Geometry: final body of the model. Coordinates: model frame, mm. Face numbers are marked on the shaded views. A direction names the side the tool comes from. Round coordinates to 2 decimals unless told otherwise and drop trailing zeros. Loops run counter-clockwise (first coordinate to the right, second up) from the corner with the lowest first, then second, coordinate; pieces in that order, holes last. Notation, with made-up numbers: (7, 21) -> (46, 21) arc R9 cw to (46, 27) -> close; hole circle Ø1 at (18.25, 61.25). An arc over 180 degrees is marked (long way). Answer in a Markdown table with one row per item.
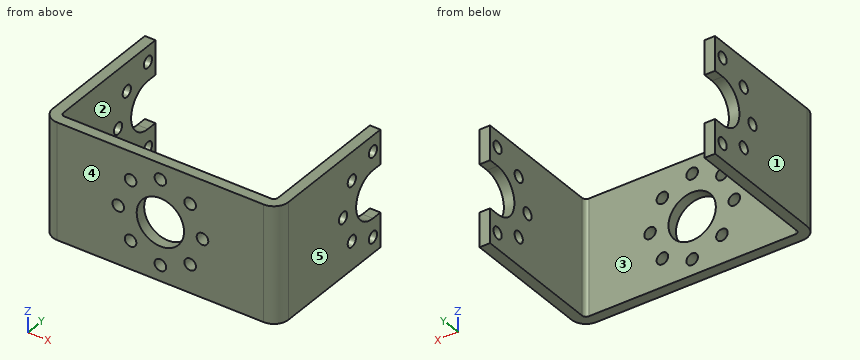
```python
from build123d import *

# Parameters (mm, degrees)
SKETCH_1_R             = 4.5
SKETCH_1_R_2           = 1.1
SM_BASE_FLANGE_1_DEPTH = 2
OTHER_START            = -47
OTHER_1_OUTLINE_W      = 2
OTHER_1_OUTLINE_H      = 22
OTHER_1_DEPTH          = 24.627322451
OTHER_START_2          = 22.372677549
OTHER_1_2_OUTLINE_W    = 2
OTHER_1_2_OUTLINE_H    = 22
OTHER_1_2_DEPTH        = 24.627322451
OTHER_START_3          = -22.106515833
OTHER_1_3_OUTLINE_R    = 1.1
OTHER_1_3_DEPTH        = 1.733838284
OTHER_START_4          = 20.372677549
OTHER_1_4_OUTLINE_R    = 1.1
OTHER_1_4_DEPTH        = 1.733838284
OTHER_START_5          = -22.372677549
OTHER_1_5_OUTLINE_R    = 1.1
OTHER_1_5_DEPTH        = 2.7366
OTHER_START_6          = 19.636077549
OTHER_1_6_OUTLINE_R    = 1.1
OTHER_1_6_DEPTH        = 2.7366
OTHER_START_7          = -12
OTHER_1_7_DEPTH        = 24


with BuildPart() as part:
    # 基体-法兰1: sheet metal written as solids
    # Sketch 1 → 基体-法兰1 (new body)
    with BuildSketch(Plane(origin=(0, 0, 0), x_dir=(1, 0, 0), z_dir=(0, 1, 0))):
        with BuildLine():
            Line((-45, -11), (-47, -11))
            Line((-47, -11), (-47, -4.5))
            Line((-47, -4.5), (-45, -4.5))
            ThreePointArc((-45, -4.5), (-40.5, 0), (-45, 4.5))
            Line((-45, 4.5), (-47, 4.5))
            Line((-47, 4.5), (-47, 11))
            Line((-47, 11), (-45, 11))
            Line((-45, 11), (45, 11))
            Line((45, 11), (47, 11))
            Line((47, 11), (47, 4.5))
            Line((47, 4.5), (45, 4.5))
            ThreePointArc((45, 4.5), (40.5, 0), (45, -4.5))
            Line((45, -4.5), (47, -4.5))
            Line((47, -4.5), (47, -11))
            Line((47, -11), (45, -11))
            Line((45, -11), (-45, -11))
        make_face()
        with Locations(Location((0, 0, 0), (0, 0, 270))):
            Circle(SKETCH_1_R, mode=Mode.SUBTRACT)
        with Locations(Location((0, 8, 0), (0, 0, 270))):
            Circle(SKETCH_1_R_2, mode=Mode.SUBTRACT)
        with Locations(Location((5.656854249, 5.656854249, 0), (0, 0, 270))):
            Circle(SKETCH_1_R_2, mode=Mode.SUBTRACT)
        with Locations(Location((8, 0, 0), (0, 0, 270))):
            Circle(SKETCH_1_R_2, mode=Mode.SUBTRACT)
        with Locations(Location((5.656854249, -5.656854249, 0), (0, 0, 270))):
            Circle(SKETCH_1_R_2, mode=Mode.SUBTRACT)
        with Locations(Location((0, -8, 0), (0, 0, 270))):
            Circle(SKETCH_1_R_2, mode=Mode.SUBTRACT)
        with Locations(Location((-5.656854249, -5.656854249, 0), (0, 0, 270))):
            Circle(SKETCH_1_R_2, mode=Mode.SUBTRACT)
        with Locations(Location((-8, 0, 0), (0, 0, 270))):
            Circle(SKETCH_1_R_2, mode=Mode.SUBTRACT)
        with Locations(Location((-5.656854249, 5.656854249, 0), (0, 0, 270))):
            Circle(SKETCH_1_R_2, mode=Mode.SUBTRACT)
        with Locations(Location((-45, 8, 0), (0, 0, 270))):
            Circle(SKETCH_1_R_2, mode=Mode.SUBTRACT)
        with Locations(Location((-39.343145751, 5.656854249, 0), (0, 0, 270))):
            Circle(SKETCH_1_R_2, mode=Mode.SUBTRACT)
        with Locations(Location((-37, 0, 0), (0, 0, 270))):
            Circle(SKETCH_1_R_2, mode=Mode.SUBTRACT)
        with Locations(Location((-39.343145751, -5.656854249, 0), (0, 0, 270))):
            Circle(SKETCH_1_R_2, mode=Mode.SUBTRACT)
        with Locations(Location((-45, -8, 0), (0, 0, 270))):
            Circle(SKETCH_1_R_2, mode=Mode.SUBTRACT)
        with Locations(Location((45, 8, 0), (0, 0, 270))):
            Circle(SKETCH_1_R_2, mode=Mode.SUBTRACT)
        with Locations(Location((45, -8, 0), (0, 0, 270))):
            Circle(SKETCH_1_R_2, mode=Mode.SUBTRACT)
        with Locations(Location((39.343145751, -5.656854249, 0), (0, 0, 270))):
            Circle(SKETCH_1_R_2, mode=Mode.SUBTRACT)
        with Locations(Location((37, 0, 0), (0, 0, 270))):
            Circle(SKETCH_1_R_2, mode=Mode.SUBTRACT)
        with Locations(Location((39.343145751, 5.656854249, 0), (0, 0, 270))):
            Circle(SKETCH_1_R_2, mode=Mode.SUBTRACT)
    extrude(amount=-SM_BASE_FLANGE_1_DEPTH)

    # Other 1: read off the stored shape, not the designer's step
    # Other 1 outline → Other 1 (cut)
    with BuildSketch(Plane.YZ.offset(OTHER_START)):
        with Locations((-1, 0)):
            Rectangle(OTHER_1_OUTLINE_W, OTHER_1_OUTLINE_H)
    extrude(amount=OTHER_1_DEPTH, mode=Mode.SUBTRACT)

    # Other 1 2 outline → Other 1 2 (cut)
    with BuildSketch(Plane.YZ.offset(OTHER_START_2)):
        with Locations((-1, 0)):
            Rectangle(OTHER_1_2_OUTLINE_W, OTHER_1_2_OUTLINE_H)
    extrude(amount=OTHER_1_2_DEPTH, mode=Mode.SUBTRACT)

    # Other 1 3 outline → Other 1 3 (add)
    with BuildSketch(Plane.YZ.offset(OTHER_START_3)):
        with BuildLine():
            Line((0, 11), (0, -11))
            Line((0, -11), (25.372677549, -11))
            Line((25.372677549, -11), (25.372677549, -4.5))
            Line((25.372677549, -4.5), (23.372677549, -4.5))
            ThreePointArc((23.372677549, -4.5), (18.872677549, 0), (23.372677549, 4.5))
            Line((23.372677549, 4.5), (25.372677549, 4.5))
            Line((25.372677549, 4.5), (25.372677549, 11))
            Line((25.372677549, 11), (0, 11))
        make_face()
        with Locations((17.7158233, -5.656854249)):
            Circle(OTHER_1_3_OUTLINE_R, mode=Mode.SUBTRACT)
        with Locations((23.372677549, -8)):
            Circle(OTHER_1_3_OUTLINE_R, mode=Mode.SUBTRACT)
        with Locations((15.372677549, 0)):
            Circle(OTHER_1_3_OUTLINE_R, mode=Mode.SUBTRACT)
        with Locations((17.7158233, 5.656854249)):
            Circle(OTHER_1_3_OUTLINE_R, mode=Mode.SUBTRACT)
        with Locations((23.372677549, 8)):
            Circle(OTHER_1_3_OUTLINE_R, mode=Mode.SUBTRACT)
    extrude(amount=OTHER_1_3_DEPTH)

    # Other 1 4 outline → Other 1 4 (add)
    with BuildSketch(Plane.YZ.offset(OTHER_START_4)):
        with BuildLine():
            Line((0, 11), (0, -11))
            Line((0, -11), (25.372677549, -11))
            Line((25.372677549, -11), (25.372677549, -4.5))
            Line((25.372677549, -4.5), (23.372677549, -4.5))
            ThreePointArc((23.372677549, -4.5), (18.872677549, 0), (23.372677549, 4.5))
            Line((23.372677549, 4.5), (25.372677549, 4.5))
            Line((25.372677549, 4.5), (25.372677549, 11))
            Line((25.372677549, 11), (0, 11))
        make_face()
        with Locations((17.7158233, -5.656854249)):
            Circle(OTHER_1_4_OUTLINE_R, mode=Mode.SUBTRACT)
        with Locations((23.372677549, -8)):
            Circle(OTHER_1_4_OUTLINE_R, mode=Mode.SUBTRACT)
        with Locations((15.372677549, 0)):
            Circle(OTHER_1_4_OUTLINE_R, mode=Mode.SUBTRACT)
        with Locations((17.7158233, 5.656854249)):
            Circle(OTHER_1_4_OUTLINE_R, mode=Mode.SUBTRACT)
        with Locations((23.372677549, 8)):
            Circle(OTHER_1_4_OUTLINE_R, mode=Mode.SUBTRACT)
    extrude(amount=OTHER_1_4_DEPTH)

    # Other 1 5 outline → Other 1 5 (add)
    with BuildSketch(Plane.YZ.offset(OTHER_START_5)):
        with BuildLine():
            Line((0, -11), (25.372677549, -11))
            Line((25.372677549, -11), (25.372677549, -4.5))
            Line((25.372677549, -4.5), (23.372677549, -4.5))
            ThreePointArc((23.372677549, -4.5), (18.872677549, 0), (23.372677549, 4.5))
            Line((23.372677549, 4.5), (25.372677549, 4.5))
            Line((25.372677549, 4.5), (25.372677549, 11))
            Line((25.372677549, 11), (0, 11))
            Line((0, 11), (0, -11))
        make_face()
        with Locations((17.7158233, -5.656854249)):
            Circle(OTHER_1_5_OUTLINE_R, mode=Mode.SUBTRACT)
        with Locations((23.372677549, -8)):
            Circle(OTHER_1_5_OUTLINE_R, mode=Mode.SUBTRACT)
        with Locations((15.372677549, 0)):
            Circle(OTHER_1_5_OUTLINE_R, mode=Mode.SUBTRACT)
        with Locations((17.7158233, 5.656854249)):
            Circle(OTHER_1_5_OUTLINE_R, mode=Mode.SUBTRACT)
        with Locations((23.372677549, 8)):
            Circle(OTHER_1_5_OUTLINE_R, mode=Mode.SUBTRACT)
    extrude(amount=OTHER_1_5_DEPTH)

    # Other 1 6 outline → Other 1 6 (add)
    with BuildSketch(Plane.YZ.offset(OTHER_START_6)):
        with BuildLine():
            Line((0, -11), (25.372677549, -11))
            Line((25.372677549, -11), (25.372677549, -4.5))
            Line((25.372677549, -4.5), (23.372677549, -4.5))
            ThreePointArc((23.372677549, -4.5), (18.872677549, 0), (23.372677549, 4.5))
            Line((23.372677549, 4.5), (25.372677549, 4.5))
            Line((25.372677549, 4.5), (25.372677549, 11))
            Line((25.372677549, 11), (0, 11))
            Line((0, 11), (0, -11))
        make_face()
        with Locations((17.7158233, -5.656854249)):
            Circle(OTHER_1_6_OUTLINE_R, mode=Mode.SUBTRACT)
        with Locations((23.372677549, -8)):
            Circle(OTHER_1_6_OUTLINE_R, mode=Mode.SUBTRACT)
        with Locations((15.372677549, 0)):
            Circle(OTHER_1_6_OUTLINE_R, mode=Mode.SUBTRACT)
        with Locations((17.7158233, 5.656854249)):
            Circle(OTHER_1_6_OUTLINE_R, mode=Mode.SUBTRACT)
        with Locations((23.372677549, 8)):
            Circle(OTHER_1_6_OUTLINE_R, mode=Mode.SUBTRACT)
    extrude(amount=OTHER_1_6_DEPTH)

    # Other 1 7 outline → Other 1 7 (cut)
    with BuildSketch(Plane.XY.offset(OTHER_START_7)):
        with BuildLine():
            Line((-22.372677549, -2), (-19.636077549, -2))
            ThreePointArc((-19.636077549, -2), (-21.571145966, -1.198468418), (-22.372677549, 0.7366))
            Line((-22.372677549, 0.7366), (-22.372677549, -2))
        make_face()
        with BuildLine():
            Line((20.372677549, 0.7366), (20.372677549, 25.372677549))
            Line((20.372677549, 25.372677549), (19.636077549, 25.372677549))
            Line((19.636077549, 25.372677549), (19.636077549, 0))
            ThreePointArc((19.636077549, 0), (20.156932404, 0.215745145), (20.372677549, 0.7366))
        make_face()
        with BuildLine():
            ThreePointArc((22.372677549, 0.7366), (21.571145966, -1.198468418), (19.636077549, -2))
            Line((19.636077549, -2), (22.372677549, -2))
            Line((22.372677549, -2), (22.372677549, 0.7366))
        make_face()
        with BuildLine():
            Line((-19.636077549, 25.372677549), (-20.372677549, 25.372677549))
            Line((-20.372677549, 25.372677549), (-20.372677549, 0.7366))
            ThreePointArc((-20.372677549, 0.7366), (-20.156932404, 0.215745145), (-19.636077549, 0))
            Line((-19.636077549, 0), (-19.636077549, 25.372677549))
        make_face()
    extrude(amount=OTHER_1_7_DEPTH, mode=Mode.SUBTRACT)


solid = part.part
```
Item 1: Section query B-B, the plane x = 8. Output: boundary loops of the cut face in (y, z).
Ans:
| item | result |
|---|---|
| outline | (-2, -11) -> (0, -11) -> (0, -1.1) -> (-2, -1.1) -> close; (-2, 1.1) -> (0, 1.1) -> (0, 11) -> (-2, 11) -> close |
Item 2: Mould query, pull axis X, two halves, no side actions, for the marked faces 3, 4 and 5. Classes: released by +X, released by -X, zero draft, split by the parting line, or undercut.
Ans:
| item | result |
|---|---|
| face 3 | undercut |
| face 4 | zero draft |
| face 5 | released by +X |
Item 3: First-contact query: P1, Ø8, axis at x = -3, z = -1, coming from the -Y side. Flat tip, straight axial feed; report the tip coordinate or a pass-through.
Ans:
| item | result |
|---|---|
| P1 | y = -2 |
Item 4: Set-up query: the marked faces 1 and 2. Return all of +Z, -Z, +X, -X, +Y, -Y with unobstructed straight access to the full face (end or side cutting, diameter ignored); none if empty.
Ans:
| item | result |
|---|---|
| face 1 | +Z, -Z, -X, +Y, -Y |
| face 2 | +Z, -Z, +Y |
Item 5: Section query C-C, the plane z = 8. Output: boundary loops of the cut face in (x, y), and give its area (3 significant figures).
Ans:
| item | result |
|---|---|
| outline | (-22.37, 0.74) arc R2.74 ccw to (-19.64, -2) -> (-1.1, -2) -> (-1.1, 0) -> (-19.64, 0) arc R0.74 cw to (-20.37, 0.74) -> (-20.37, 22.27) -> (-22.37, 22.27) -> close; (-22.37, 24.47) -> (-20.37, 24.47) -> (-20.37, 25.37) -> (-22.37, 25.37) -> close; (1.1, -2) -> (19.64, -2) arc R2.74 ccw to (22.37, 0.74) -> (22.37, 22.27) -> (20.37, 22.27) -> (20.37, 0.74) arc R0.74 cw to (19.64, 0) -> (1.1, 0) -> close; (20.37, 24.47) -> (22.37, 24.47) -> (22.37, 25.37) -> (20.37, 25.37) -> close |
| area | 175 mm2 |
Item 6: Section query D-D, the plane x = 0. Output: boundary loops of the cut face in (y, z).
Ans:
| item | result |
|---|---|
| outline | (-2, -11) -> (0, -11) -> (0, -9.1) -> (-2, -9.1) -> close; (-2, -6.9) -> (0, -6.9) -> (0, -4.5) -> (-2, -4.5) -> close; (-2, 4.5) -> (0, 4.5) -> (0, 6.9) -> (-2, 6.9) -> close; (-2, 9.1) -> (0, 9.1) -> (0, 11) -> (-2, 11) -> close |
Item 7: Ray query, L1, parallel to X at y = 22.25, z = 10; L2, parallel to X at y = -0.5, z = -4.75; L3, parallel to Y at x = 17, z = 8. Return the intervals inside material, ascending.
Ans:
| item | result |
|---|---|
| L1 | -22.37 to -20.37, 20.37 to 22.37 |
| L2 | -22.08 to -6.28, -5.03 to 5.03, 6.28 to 22.08 |
| L3 | -2 to 0 |
Item 8: Section query A-A, the plane y = 3.5. Output: boundary loops of the cut face in (x, z).
Ans:
| item | result |
|---|---|
| outline | (-22.37, -11) -> (-20.37, -11) -> (-20.37, 11) -> (-22.37, 11) -> close; (20.37, -11) -> (22.37, -11) -> (22.37, 11) -> (20.37, 11) -> close |
